Verification items for the finished model (mm, model axes). A direction names the side the tool comes from. Round coordinates to 2 decimals unless told otherwise and drop trailing zeros. Loops run counter-clockwise (first coordinate to the right, second up) from the corner with the lowest first, then second, coordinate; pieces in that order, holes last. Notation, with made-up numbers: (-16, -24.75) - (-6, -24.75) arc R23 cw to (-6, -7.75) - close; hole circle Ø6 at (10.5, 61). An arc over 180 degrees is marked (long way). Use CSV: the item, a comma, the result in double quotes.
```python
from build123d import *

# Parameters (mm, degrees)
F0_R     = 11
F0_R_2   = 4
F1_DEPTH = 7
F2_R     = 10
F2_R_2   = 5
F3_DEPTH = 0.5
F4_R     = 10
F4_R_2   = 5
F5_DEPTH = 0.5
F6_R     = 0.2


with BuildPart() as f1:
    # F0 (on Top) → F1 (new body)
    with BuildSketch(Plane.XY):
        Circle(F0_R)
        Circle(F0_R_2, mode=Mode.SUBTRACT)
    extrude(amount=F1_DEPTH)

    # F2 (on face) → F3 (cut)
    with BuildSketch(Plane(origin=(0, 0, 0), x_dir=(1, 0, 0), z_dir=(0, 0, -1))):
        Circle(F2_R)
        Circle(F2_R_2, mode=Mode.SUBTRACT)
    extrude(amount=-F3_DEPTH, mode=Mode.SUBTRACT)

    # F4 (on face) → F5 (cut)
    with BuildSketch(Plane.XY.offset(7)):
        Circle(F4_R)
        Circle(F4_R_2, mode=Mode.SUBTRACT)
    extrude(amount=-F5_DEPTH, mode=Mode.SUBTRACT)

    # F6
    f6_edges = [f1.edges().sort_by_distance(p)[0] for p in [
        (-11, 0, 0),
        (-11, 0, 7),
    ]]
    fillet(f6_edges, radius=F6_R)


solid = f1.part
```
1) Access from +Z, -Z, +X, -X, +Y, -Y to the whole of each face (thin tool, end or side, straight path). Record for faces 1 (the face through (3, -10, 7)), 2 (the face through (-5, 2, 0.5)), 3 (the face through (-2.17, -9.76, 6.75)).
Returned:
face 1,"+Z, +X, -X, +Y, -Y"
face 2,"-Z"
face 3,"+Z"
2) Mould release check, pull along X, two halves, no side actions. Record for faces 4 (the face through (3, -10, 0)), 5 (the face through (-2.38, -10.74, 3.45)), 6 (the face through (-0.867, -3.905, 3.451)): +X half, -X half, draft (parallel to the pull), parting line (faces both ways), or undercut.
Returned:
face 4,"draft"
face 5,"parting line"
face 6,"undercut"
3) Gauge pin test, flat ends, axial feed: pin 1 Ø1 at (x, z) = (1.5, 5) entering from +Y; pin 2 Ø1 at (x, z) = (-6, 4) entering from +Y; pin 3 Ø1.5 at (x, z) = (-4.5, 4.5) entering from -Y. Record the tip position at first contact, or that the pin passes through.
Returned:
pin 1,"stops at y = 10.95"
pin 2,"stops at y = 9.53"
pin 3,"stops at y = -10.34"
4) Cross-section at B-B, the plane z = 4. Record the cut outline in (x, y).
Returned:
outline,"circle Ø22 at (0, 0); hole circle Ø8 at (0, 0)"
5) Thickness scan on probe 1 along Y at (x, z) = (0, 6.65); probe 2 along Y at (x, z) = (0, 4.25); probe 3 along X at (y, z) = (2, 3.5). Record the ranges inside material, lowest first. Write a range as [from, to].
Returned:
probe 1,"y = [-11, -10], [-5, -4], [4, 5], [10, 11]"
probe 2,"y = [-11, -4], [4, 11]"
probe 3,"x = [-10.82, -3.46], [3.46, 10.82]"
6) Cross-section at A-A, the plane y = 0. Record the cut outline in (x, z), then the cut area to 3 significant figures.
Returned:
outline,"(-11, 0.2) arc R0.2 ccw to (-10.8, 0) - (-10, 0) - (-10, 0.5) - (-5, 0.5) - (-5, 0) - (-4, 0) - (-4, 7) - (-5, 7) - (-5, 6.5) - (-10, 6.5) - (-10, 7) - (-10.8, 7) arc R0.2 ccw to (-11, 6.8) - close; (4, 0) - (5, 0) - (5, 0.5) - (10, 0.5) - (10, 0) - (10.8, 0) arc R0.2 ccw to (11, 0.2) - (11, 6.8) arc R0.2 ccw to (10.8, 7) - (10, 7) - (10, 6.5) - (5, 6.5) - (5, 7) - (4, 7) - close"
area,"88.0 mm²"
